Read the model definition and answer for the solid it produces. Units are mm, in the model's axes. Round coordinates to 2 decimals unless told otherwise and drop trailing zeros. Order: outer loops, then holes, each group sorted by start corner. A loop starts at its lowest first (then second) coordinate and runs counter-clockwise, first axis right, second up. Notation, with made-up numbers: (36.25, 74) -> (92.25, 74) arc R31 ccw to (92.25, 109) -> close; hole circle Ø5 at (-22.75, 65). An arc over 180 degrees is marked (long way). One line per item, written item: value. Start each with the question number.
1. Consider line 1 (Y direction, x = 0, z = 0); line 2 (Y direction, x = 10, z = 0.65); line 3 (Y direction, x = -9, z = 0.75). Determine where each line is inside the solid, lowest interval first.
2. Section D-D (z = 0.35) is taken. State how many separate pieces and enclosed holes the cut face has, then the cut area to 3 significant figures.
3. Section C-C (y = 50) is taken. Give the vertices of the cut face in (x, z).
4. Flat-ended cylindrical pins translate along their axes: pin 1 Ø1.5 at (y, z) = (8.5, -0.5) entering from +X; pin 2 Ø2 at (x, y) = (50, 0) entering from -Z; pin 3 Ø1.5 at (y, z) = (27, -0.5) entering from -X; pin 4 Ø4.5 at (x, y) = (8.84, 8.84) entering from +Z. Find the tip coordinate at first contact, or state that the pin passes through.
5. Section B-B (x = -40) is taken. Give the vertices of the cut face in (y, z), then the cut area to 3 significant figures.
6. Section A-A (y = 0) is taken. Give the vertices of the cut face in (x, z).
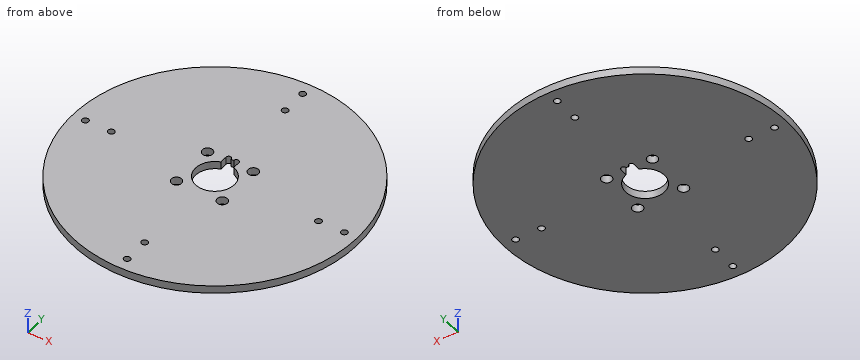
from build123d import *

# Parameters (mm, degrees)
SKETCH_1_R               = 55
EXTRUDE_1_DEPTH          = 1.5
CUT_EXTRUDE_7_DEPTH      = 78.796208134
CUT_EXTRUDE_7_DEPTH_BACK = 78.796208134
M3X0_5_1_D               = 2.5
F_4_0MM_1_D              = 4
F_4_0MM_1_DEPTH          = 5
F_4_0MM_1_TIP            = 1.201721238


with BuildPart() as part:
    # Sketch 1 → Extrude 1 (new, symmetric)
    with BuildSketch(Plane.XY):
        Circle(SKETCH_1_R)
    extrude(amount=EXTRUDE_1_DEPTH, both=True)

    # Sketch 1_4 → Cut-Extrude 7 (cut, two sides: drawn at the far end of the back side and taken through both)
    with BuildSketch(Plane.XY.offset(-CUT_EXTRUDE_7_DEPTH_BACK)):
        with BuildLine():
            ThreePointArc((-2.5, 10), (-1.5, 11), (-0.5, 10))
            Line((-0.5, 10), (0.5, 10))
            ThreePointArc((0.5, 10), (1.5, 11), (2.5, 10))
            Line((2.5, 10), (2.5, 7.071067812))
            ThreePointArc((2.5, 7.071067812), (0, -7.5), (-2.5, 7.071067812))
            Line((-2.5, 7.071067812), (-2.5, 10))
        make_face()
    extrude(amount=CUT_EXTRUDE_7_DEPTH + CUT_EXTRUDE_7_DEPTH_BACK, mode=Mode.SUBTRACT)

    # M3x0.5 _1 (through all)
    with Locations(Plane(origin=(0, 50, 1.5), x_dir=(1, 0, 0), z_dir=(0, 0, 1))):
        with Locations((0, 0), (0, -10), (-50, -50), (-40, -50), (0, -100), (0, -90), (50, -50), (40, -50)):
            Hole(M3X0_5_1_D / 2)

    # 4.0mm _1
    with Locations(Plane.XY.offset(1.5)):
        with Locations((-8.838834765, -8.838834765), (-8.838834765, 8.838834765), (8.838834765, 8.838834765), (8.838834765, -8.838834765)):
            Hole(F_4_0MM_1_D / 2, depth=F_4_0MM_1_DEPTH)
            with Locations((0, 0, -(F_4_0MM_1_DEPTH + F_4_0MM_1_TIP / 2))):  # 118° drill point
                Cone(0, F_4_0MM_1_D / 2, F_4_0MM_1_TIP, mode=Mode.SUBTRACT)


solid = part.part
Answer:
1. line 1: -55 to -51.25, -48.75 to -41.25, -38.75 to -7.5, 10 to 38.75, 41.25 to 48.75, 51.25 to 55
1. line 2: -54.08 to -10.47, -7.21 to 7.21, 10.47 to 54.08
1. line 3: -54.26 to -10.83, -6.85 to 6.85, 10.83 to 54.26
2. separate pieces: 1
2. enclosed holes: 13
2. area: 9,220 mm^2
3. outline: (-22.91, -1.5) -> (-1.25, -1.5) -> (-1.25, 1.5) -> (-22.91, 1.5) -> close; (1.25, -1.5) -> (22.91, -1.5) -> (22.91, 1.5) -> (1.25, 1.5) -> close
4. pin 1: x = 54.45
4. pin 2: through
4. pin 3: x = -48.33
4. pin 4: z = 1.5
5. outline: (-37.75, -1.5) -> (-1.25, -1.5) -> (-1.25, 1.5) -> (-37.75, 1.5) -> close; (1.25, -1.5) -> (37.75, -1.5) -> (37.75, 1.5) -> (1.25, 1.5) -> close
5. area: 219 mm^2
6. outline: (-55, -1.5) -> (-51.25, -1.5) -> (-51.25, 1.5) -> (-55, 1.5) -> close; (-48.75, -1.5) -> (-41.25, -1.5) -> (-41.25, 1.5) -> (-48.75, 1.5) -> close; (-38.75, -1.5) -> (-7.5, -1.5) -> (-7.5, 1.5) -> (-38.75, 1.5) -> close; (7.5, -1.5) -> (38.75, -1.5) -> (38.75, 1.5) -> (7.5, 1.5) -> close; (41.25, -1.5) -> (48.75, -1.5) -> (48.75, 1.5) -> (41.25, 1.5) -> close; (51.25, -1.5) -> (55, -1.5) -> (55, 1.5) -> (51.25, 1.5) -> close
